from build123d import *

# Parameters (mm, degrees)
SKETCH1_R           = 2.5
BOSS_EXTRUDE1_DEPTH = 5
SKETCH2_R           = 10
SKETCH2_R_2         = 2.5
BOSS_EXTRUDE2_DEPTH = 5
SKETCH3_W           = 2.5
SKETCH3_H           = 5.7
CUT_EXTRUDE1_DEPTH  = 5
SKETCH4_R           = 1.65
CUT_EXTRUDE2_DEPTH  = 25


with BuildPart() as part:
    # Sketch1 → Boss-Extrude1 (new body)
    with BuildSketch(Plane(origin=(0, 0, 0), x_dir=(1, 0, 0), z_dir=(0, 1, 0))):
        with BuildLine():
            ThreePointArc((-21.5, -7.5), (-11.330511131, -9.033592317), (-1.086131732, -9.940840903))
            ThreePointArc((-1.086131732, -9.940840903), (-0.543113838, -9.971301197), (0, -10))
            ThreePointArc((0, -10), (10, 0), (0, 10))
            ThreePointArc((0, 10), (-0.543113838, 9.971301197), (-1.086131732, 9.940840903))
            ThreePointArc((-1.086131732, 9.940840903), (-11.330511131, 9.033592317), (-21.5, 7.5))
            ThreePointArc((-21.5, 7.5), (-29, 0), (-21.5, -7.5))
        make_face()
        with Locations(Location((0, 0, 0), (0, 0, 270))):
            Circle(SKETCH1_R, mode=Mode.SUBTRACT)
    extrude(amount=BOSS_EXTRUDE1_DEPTH)

    # Sketch2 → Boss-Extrude2 (add)
    with BuildSketch(Plane(origin=(0, 5, 0), x_dir=(1, 0, 0), z_dir=(0, 1, 0))):
        with Locations(Location((0, 0, 0), (0, 0, 270))):
            Circle(SKETCH2_R)
        with Locations(Location((0, 0, 0), (0, 0, 270))):
            Circle(SKETCH2_R_2, mode=Mode.SUBTRACT)
    extrude(amount=BOSS_EXTRUDE2_DEPTH)

    # Sketch3 → Cut-Extrude1 (cut)
    with BuildSketch(Plane(origin=(0, 10, 0), x_dir=(1, 0, 0), z_dir=(0, 1, 0))):
        with Locations((6.25, 0)):
            Rectangle(SKETCH3_W, SKETCH3_H)
    extrude(amount=-CUT_EXTRUDE1_DEPTH, mode=Mode.SUBTRACT)

    # Sketch4 → Cut-Extrude2 (cut)
    with BuildSketch(Plane(origin=(0, 0, 0), x_dir=(0, 0, -1), z_dir=(1, 0, 0))):
        with Locations(Location((0, 7.5, 0), (0, 0, 180))):
            Circle(SKETCH4_R)
    extrude(amount=CUT_EXTRUDE2_DEPTH, mode=Mode.SUBTRACT)


solid = part.part
CAD build for the part. Positions are in the model's coordinates, mm. A direction names the side the tool comes from. Round coordinates to 2 decimals unless told otherwise and drop trailing zeros. Loops run counter-clockwise (first coordinate to the right, second up) from the corner with the lowest first, then second, coordinate; pieces in that order, holes last.
(1) Cut at D-D (x = -2). Give the cut face in (y, z), plus the area to 3 significant figures.
(2) Cut at C-C (z = 8.5). Give the cut face in (x, y).
(3) Cut at B-B (x = 6.5). Give the cut face in (y, z), plus the area to 3 significant figures.
(4) Drop flat-ended pins along their axis: pin 1 (3 mm diameter, centred on x = 6, y = 6.5, fed in from -Z); pin 2 (5 mm diameter, centred on x = -8, y = 1, fed in from +Z); pin 3 (6 mm diameter, centred on y = 8.5, z = 4, fed in from -X); pin 4 (1.5 mm diameter, centred on x = -23.5, y = 7.5, fed in from -Z). Give the stop position or say it passes through.
(5) Wall check: line 1 along Y through (x, z) = (8.55, 0); line 2 along X through (y, z) = (5.25, 0); line 3 along X through (y, z) = (9.25, -0.75). Give the ranges that are in metal, low to high.
(6) Cut at A-A (y = 1). Give the cut face in (x, z), plus the area to 3 significant figures.
(7) Which spindle directions (+Z, -Z, +X, -X, +Y, -Y) get a long thin tool onto all of the face, cutting with end or side? Do faces 1 (the flat face through (7.5, 9, 1)), 2 (the cylindrical face through (8.7, 9.1, -0.4)), 3 (the cylindrical face through (-29, 2, 0)). Say none if no direction does.
(8) Two-plate mould, pull along X, no slides. Class faces 4 (the flat face through (6, 5, 0)), 5 (the cylindrical face through (9.915, 6.041, -1.302)), 6 (the cylindrical face through (3.42, 6.11, 0.89)): +X half, -X half, draft (parallel to the pull), parting line (faces both ways), or undercut.
Findings below:
1. outline: (0, -9.89) - (5, -9.89) - (5, -9.8) - (10, -9.8) - (10, -1.5) - (0, -1.5) - close; (0, 1.5) - (10, 1.5) - (10, 9.8) - (5, 9.8) - (5, 9.89) - (0, 9.89) - close
1. area: 167 mm2
2. outline: (-15.38, 0) - (5.27, 0) - (5.27, 10) - (-5.27, 10) - (-5.27, 5) - (-15.38, 5) - close
3. outline: (0, -7.6) - (10, -7.6) - (10, -2.85) - (5, -2.85) - (5, 2.85) - (10, 2.85) - (10, 7.6) - (0, 7.6) - close
3. area: 123 mm2
4. pin 1: stops at z = -8.93
4. pin 2: stops at z = 9.63
4. pin 3: stops at x = -9.95
4. pin 4: passes through
5. line 1: y = 0 to 5.85, 9.15 to 10
5. line 2: x = -10 to -2.5, 2.5 to 5, 7.5 to 10
5. line 3: x = -9.97 to -2.38, 2.38 to 5, 7.5 to 9.97
6. outline: (-21.5, -7.5) arc R167.68 ccw to (0, -10) arc R10 ccw to (0, 10) arc R167.68 ccw to (-21.5, 7.5) arc R7.5 ccw to start; hole circle Ø5 at (0, 0)
6. area: 612 mm2
7. face 1: +Y
7. face 2: +X
7. face 3: -X, +Y, -Y
8. face 4: undercut
8. face 5: parting line
8. face 6: draft
